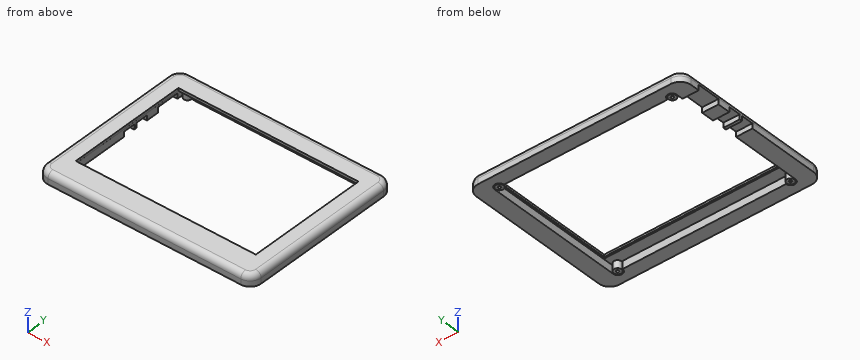
from build123d import *

# Parameters (mm, degrees)
BOSS_EXTRU_1_DEPTH      = 10
ESQUISSE2_W             = 163.5
ESQUISSE2_H             = 109
ENL_V_MAT_EXTRU_1_DEPTH = 10
ESQUISSE3_W             = 164.5
ESQUISSE3_H             = 110
ENL_V_MAT_EXTRU_2_DEPTH = 8
ENL_V_MAT_EXTRU_3_DEPTH = 7
ESQUISSE5_R             = 3.5
ESQUISSE5_R_2           = 1.25
BOSS_EXTRU_2_DEPTH      = 7
CONG_1_R                = 5
ESQUISSE6_W             = 12.13
ESQUISSE6_H             = 21
ESQUISSE6_W_2           = 8
ESQUISSE6_H_2           = 11
ENL_V_MAT_EXTRU_4_DEPTH = 97.5


with BuildPart() as part:
    # Esquisse1 → Boss.-Extru.1 (new body)
    with BuildSketch(Plane.XY):
        with BuildLine():
            Line((87.5, -75), (-87.5, -75))
            ThreePointArc((-87.5, -75), (-94.571067812, -72.071067812), (-97.5, -65))
            Line((-97.5, -65), (-97.5, 65))
            ThreePointArc((-97.5, 65), (-94.571067812, 72.071067812), (-87.5, 75))
            Line((-87.5, 75), (87.5, 75))
            ThreePointArc((87.5, 75), (94.571067812, 72.071067812), (97.5, 65))
            Line((97.5, 65), (97.5, -65))
            ThreePointArc((97.5, -65), (94.571067812, -72.071067812), (87.5, -75))
        make_face()
    extrude(amount=BOSS_EXTRU_1_DEPTH)

    # Esquisse2 → Enlèv. mat.-Extru.1 (cut)
    with BuildSketch(Plane.XY.offset(10)):
        with Locations((0, 2.25)):
            Rectangle(ESQUISSE2_W, ESQUISSE2_H)
    extrude(amount=-ENL_V_MAT_EXTRU_1_DEPTH, mode=Mode.SUBTRACT)

    # Esquisse3 → Enlèv. mat.-Extru.2 (cut)
    with BuildSketch(Plane(origin=(0, 0, 0), x_dir=(-1, 0, 0), z_dir=(0, 0, -1))):
        with Locations((0, 2.25)):
            Rectangle(ESQUISSE3_W, ESQUISSE3_H)
    extrude(amount=-ENL_V_MAT_EXTRU_2_DEPTH, mode=Mode.SUBTRACT)

    # Esquisse4 → Enlèv. mat.-Extru.3 (cut)
    with BuildSketch(Plane(origin=(0, 0, 0), x_dir=(-1, 0, 0), z_dir=(0, 0, -1))):
        with BuildLine():
            Line((-74.305753882, -63.01), (74.305753882, -63.01))
            ThreePointArc((74.305753882, -63.01), (78.51, -67.214246118), (82.714246118, -63.01))
            Line((82.714246118, -63.01), (82.714246118, 63.01))
            ThreePointArc((82.714246118, 63.01), (78.51, 67.214246118), (74.305753882, 63.01))
            Line((74.305753882, 63.01), (-74.305753882, 63.01))
            ThreePointArc((-74.305753882, 63.01), (-78.51, 67.214246118), (-82.714246118, 63.01))
            Line((-82.714246118, 63.01), (-82.714246118, -63.01))
            ThreePointArc((-82.714246118, -63.01), (-78.51, -67.214246118), (-74.305753882, -63.01))
        make_face()
    extrude(amount=-ENL_V_MAT_EXTRU_3_DEPTH, mode=Mode.SUBTRACT)

    # Esquisse5 → Boss.-Extru.2 (add)
    # profile 1 of 4: a face of its own
    with BuildSketch(Plane(origin=(0, 0, 7), x_dir=(-1, 0, 0), z_dir=(0, 0, -1))):
        with Locations(Location((-78.5, -62.75, 0), (0, 0, 180))):
            Circle(ESQUISSE5_R)
        with Locations(Location((-78.5, -62.75, 0), (0, 0, 180))):
            Circle(ESQUISSE5_R_2, mode=Mode.SUBTRACT)
    # profile 2 of 4: a face of its own
    with BuildSketch(Plane(origin=(0, 0, 7), x_dir=(-1, 0, 0), z_dir=(0, 0, -1))):
        with Locations(Location((78.5, -62.75, 0), (0, 0, 180))):
            Circle(ESQUISSE5_R)
        with Locations(Location((78.5, -62.75, 0), (0, 0, 180))):
            Circle(ESQUISSE5_R_2, mode=Mode.SUBTRACT)
    # profile 3 of 4: a face of its own
    with BuildSketch(Plane(origin=(0, 0, 7), x_dir=(-1, 0, 0), z_dir=(0, 0, -1))):
        with Locations(Location((78.5, 62.75, 0), (0, 0, 180))):
            Circle(ESQUISSE5_R)
        with Locations(Location((78.5, 62.75, 0), (0, 0, 180))):
            Circle(ESQUISSE5_R_2, mode=Mode.SUBTRACT)
    # profile 4 of 4: a face of its own
    with BuildSketch(Plane(origin=(0, 0, 7), x_dir=(-1, 0, 0), z_dir=(0, 0, -1))):
        with Locations(Location((-78.5, 62.75, 0), (0, 0, 180))):
            Circle(ESQUISSE5_R)
        with Locations(Location((-78.5, 62.75, 0), (0, 0, 180))):
            Circle(ESQUISSE5_R_2, mode=Mode.SUBTRACT)
    extrude(amount=BOSS_EXTRU_2_DEPTH)

    # Congé1
    cong_1_edges = [part.edges().sort_by_distance(p)[0] for p in [
        (-94.571067812, 72.071067812, 10),
        (-97.5, 0, 10),
        (-94.571067812, -72.071067812, 10),
        (0, -75, 10),
        (94.571067812, -72.071067812, 10),
        (97.5, 0, 10),
        (94.571067812, 72.071067812, 10),
        (0, 75, 10),
    ]]
    fillet(cong_1_edges, radius=CONG_1_R)

    # Esquisse6 → Enlèv. mat.-Extru.4 (cut)
    with BuildSketch(Plane(origin=(0, 0, 0), x_dir=(0, 0, -1), z_dir=(1, 0, 0))):
        with Locations((1.265, 46.5)):
            Rectangle(ESQUISSE6_W, ESQUISSE6_H)
        with Locations((-0.5, 19)):
            Rectangle(ESQUISSE6_W_2, ESQUISSE6_H_2)
        with Locations((-0.5, 5.5)):
            Rectangle(ESQUISSE6_W_2, ESQUISSE6_H_2)
    extrude(amount=-ENL_V_MAT_EXTRU_4_DEPTH, mode=Mode.SUBTRACT)


solid = part.part
Can you work these out from the model? Positions are in its coordinate system, mm. Round coordinates to 2 decimals unless told otherwise and drop trailing zeros. Write each loop counter-clockwise with the first axis right and the second up, starting at its lowest first coordinate (ties: lowest second). Pieces come first, ordered by that corner, then holes. Notation, with made-up numbers: (85.5, 21) -> (90.5, 21) arc R11 ccw to (90.5, 35) -> close; hole circle Ø1 at (48.5, 21.25). An arc over 180 degrees is marked (long way). One line per question, with ' | ' between items. Start each with the question number.
1) I need wall thicknesses on line 1 (X direction, y = -62.75, z = 4.5); line 2 (Y direction, x = 78.5, z = 3.5); line 3 (Y direction, x = -79, z = 3.75). Which ranges of each line are inside material? Lowest first, please. Write a range as [from, to].
2) I'm going to push flat-ended pins straight in: P1, Ø1.6, axis at y = 6, z = 9.5, coming from the +X side; P2, Ø2, axis at x = -78.5, y = -62.75, coming from the -Z side; P3, Ø0.5, axis at x = 3, z = 7.5, coming from the +Y side. Where does each tip first touch, or does it pass through?
3) Suppose I cut it at A-A on y = 3.5. Write out the boundary of the cut face in (x, z), then the cut area to 3 significant figures.
4) Suppose I cut it at B-B on x = 72. Write out the boundary of the cut face in (y, z).
Return value:
1) line 1: x = [-97.5, -82.71], [-82, -79.75], [-77.25, -75], [75, 77.25], [79.75, 82], [82.71, 97.5] | line 2: y = [-75, -67.21], [-66.25, -64], [-61.5, -59.25], [59.25, 61.5], [64, 66.25], [67.21, 75] | line 3: y = [-75, -67.19], [-66.21, -63.9], [-61.6, -59.29], [59.29, 61.6], [63.9, 66.21], [67.19, 75]
2) P1: stops at x = 95.86 | P2: stops at z = 7 | P3: stops at y = 74.47
3) outline: (-97.5, 4.5) -> (-82.71, 4.5) -> (-82.71, 7) -> (-82.25, 7) -> (-82.25, 8) -> (-81.75, 8) -> (-81.75, 10) -> (-92.5, 10) arc R5 ccw to (-97.5, 5) -> close; (81.75, 8) -> (82.25, 8) -> (82.25, 7) -> (82.71, 7) -> (82.71, 0) -> (97.5, 0) -> (97.5, 5) arc R5 ccw to (92.5, 10) -> (81.75, 10) -> close | area: 223 mm2
4) outline: (-75, 0) -> (-63.01, 0) -> (-63.01, 7) -> (-52.75, 7) -> (-52.75, 8) -> (-52.25, 8) -> (-52.25, 10) -> (-70, 10) arc R5 ccw to (-75, 5) -> close; (56.75, 8) -> (57.25, 8) -> (57.25, 7) -> (63.01, 7) -> (63.01, 0) -> (75, 0) -> (75, 5) arc R5 ccw to (70, 10) -> (56.75, 10) -> close
